from build123d import *

# Parameters (mm, degrees)
SKETCH_1_R          = 1.5
EXTRUDE_1_DEPTH     = 90
FILLET_1_R          = 0.5
SKETCH_2_R          = 1.5
EXTRUDE_2_DEPTH     = 80
SKETCH_2_3_R        = 1.5
CUT_EXTRUDE_2_DEPTH = 10


with BuildPart() as part:
    # Sketch 1 → Extrude 1 (new body)
    with BuildSketch(Plane(origin=(0, 0, 0), x_dir=(1, 0, 0), z_dir=(0, 1, 0))):
        with Locations(Location((0, 0, 0), (0, 0, 90))):
            Circle(SKETCH_1_R)
    extrude(amount=EXTRUDE_1_DEPTH)

    # Fillet 1
    fillet_1_edges = [part.edges().sort_by_distance(p)[0] for p in [
        (0, 0, 1.5),
        (0, 90, 1.5),
    ]]
    fillet(fillet_1_edges, radius=FILLET_1_R)

    # Sketch 2 → Extrude 2 (add)
    with BuildSketch(Plane(origin=(0, 0, 0), x_dir=(1, 0, 0), z_dir=(0, 1, 0))):
        Polygon((-1.625, 2.814582562), (-3.25, 0), (-1.625, -2.814582562), (1.625, -2.814582562), (3.25, 0), (1.625, 2.814582562), align=None)
        with Locations(Location((0, 0, 0), (0, 0, 90))):
            Circle(SKETCH_2_R, mode=Mode.SUBTRACT)
    extrude(amount=EXTRUDE_2_DEPTH)

    # Sketch 2_3 → Cut-Extrude 2 (cut)
    with BuildSketch(Plane(origin=(0, 0, 0), x_dir=(1, 0, 0), z_dir=(0, 1, 0))):
        Polygon((-1.625, 2.814582562), (-3.25, 0), (-1.625, -2.814582562), (1.625, -2.814582562), (3.25, 0), (1.625, 2.814582562), align=None)
        with Locations(Location((0, 0, 0), (0, 0, 90))):
            Circle(SKETCH_2_3_R, mode=Mode.SUBTRACT)
    extrude(amount=CUT_EXTRUDE_2_DEPTH, mode=Mode.SUBTRACT)


solid = part.part
For this review, take the finished solid that the model builds, in its own axes (mm). A direction names the side the tool comes from. Round coordinates to 2 decimals unless told otherwise and drop trailing zeros. Loops run counter-clockwise (first coordinate to the right, second up) from the corner with the lowest first, then second, coordinate; pieces in that order, holes last. Notation, with made-up numbers: (-31.75, -28.75) - (-20.75, -28.75) arc R20 ccw to (-20.75, -4.75) - close; hole circle Ø7 at (24.25, 8). An arc over 180 degrees is marked (long way). One line per question, with ' | ' between items.
Q1. Take a section at A-A (x = 0). Give the boundary of the cut face in (y, z), and give its area (3 significant figures).
Taken from the geometry:
outline: (0, -1) arc R0.5 ccw to (0.5, -1.5) - (10, -1.5) - (10, -2.81) - (80, -2.81) - (80, -1.5) - (89.5, -1.5) arc R0.5 ccw to (90, -1) - (90, 1) arc R0.5 ccw to (89.5, 1.5) - (80, 1.5) - (80, 2.81) - (10, 2.81) - (10, 1.5) - (0.5, 1.5) arc R0.5 ccw to (0, 1) - close | area: 454 mm²
Q2. For line 1 along Y through (x, z) = (0, 2); line 2 along X through (y, z) = (42.5, 1.35); line 3 along Z through (x, y) = (-2, 50), list the stretches that pass through material, from the lowest coordinate up. Write a range as [from, to].
Taken from the geometry:
line 1: y = [10, 80] | line 2: x = [-2.47, 2.47] | line 3: z = [-2.17, 2.17]
Q3. Tool access review of faces 1 (the flat face through (2.449, 44.51, -1.388)), 2 (the cylindrical face through (-0.45, 5.18, -1.43)), 3 (the cylindrical face through (-0.45, 84.68, -1.43)): name each direction out of +Z, -Z, +X, -X, +Y, -Y from which nothing blocks a thin tool from reaching the whole face with its end or side.
Taken from the geometry:
face 1: -Z, +X, +Y, -Y | face 2: -Y | face 3: +Y
Q4. Take a section at B-B (y = 15.5). Give the boundary of the cut face in (x, z) (3 decimals).
Taken from the geometry:
outline: (-3.25, 0) - (-1.625, -2.815) - (1.625, -2.815) - (3.25, 0) - (1.625, 2.815) - (-1.625, 2.815) - close
Q5. For pin 1 (1 mm diameter, centred on y = 74.5, z = -1.5, fed in from -X); pin 2 (3 mm diameter, centred on y = 37.5, z = -1, fed in from -X), all flat-tipped, find the tip position at first contact; note any pin that passes through.
Taken from the geometry:
pin 1: stops at x = -2.67 | pin 2: stops at x = -3.25
